```python
from build123d import *

# Parameters (mm, degrees)
CROSSRECESS_DEPTH = 0.825
DRAFT9_ANGLE      = 30
FILLET5_R         = 0.3


with BuildPart() as part:
    # Sketch1 → Base (revolve)
    with BuildSketch(Plane.XY):
        Polygon((17, 1.5), (2.65, 1.5), (1.65, 1.5), (0.55, 2.6), (0, 2.6), (0, 0), (17, 0), align=None)
    revolve(axis=Axis((4.515812911, 0, 0), (-1, 0, 0)))

    # Sketch6 → CrossRecess (cut)
    with BuildSketch(Plane(origin=(0, 0, 0), x_dir=(0, 0, -1), z_dir=(1, 0, 0))):
        Polygon((0.32, 0.32), (0.32, 1.6), (-0.32, 1.6), (-0.32, 0.32), (-1.6, 0.32), (-1.6, -0.32), (-0.32, -0.32), (-0.32, -1.6), (0.32, -1.6), (0.32, -0.32), (1.6, -0.32), (1.6, 0.32), align=None)
    extrude(amount=CROSSRECESS_DEPTH, mode=Mode.SUBTRACT)

    # Draft9
    draft9_faces = [part.faces().sort_by_distance(p)[0] for p in [
        (0.4125, 1.6, 0),
        (0.4125, 0, 1.6),
        (0.4125, -1.6, 0),
        (0.4125, 0, -1.6),
    ]]
    draft(draft9_faces, Plane(origin=(0, 2.6, 0), x_dir=(0, 0, -1), z_dir=(-1, 0, 0)), DRAFT9_ANGLE)

    # Fillet5
    fillet5_edges = [part.edges().sort_by_distance(p)[0] for p in [
        (0.4125, 0.32, 0.32),
        (0.4125, -0.32, 0.32),
        (0.4125, -0.32, -0.32),
        (0.4125, 0.32, -0.32),
    ]]
    fillet(fillet5_edges, radius=FILLET5_R)


solid = part.part
```
Could you check a few things on this model? Use its own coordinates, in mm. A direction names the side the tool comes from. Coordinates: 2 decimals unless noted, no trailing zeros. Write each loop counter-clockwise with the first axis right and the second up, starting at its lowest first coordinate (ties: lowest second). Pieces come first, ordered by that corner, then holes. Notation, with made-up numbers: (53.25, -22.5) - (91.25, -22.5) arc R16 cw to (91.25, -16.5) - close; hole circle Ø1 at (2, 67.5). An arc over 180 degrees is marked (long way). Use a Markdown table: item, result.
Q1. Please list where these lines run through material, in increasing order: L1, parallel to Y at x = 0.75, z = -0.6; L2, parallel to X at y = 1.3, z = 0.2; L3, parallel to Y at x = 12.25, z = 0.4.
Geometry check:
| item | result |
|---|---|
| L1 | y = -2.32 to -0.32, 0.32 to 2.32 |
| L2 | x = 0.52 to 17 |
| L3 | y = -1.45 to 1.45 |
Q2. Imagine slicing it at C-C (x = 2.75). List the corners of the cut face in (y, z) for me, and give its area (3 significant figures).
Geometry check:
| item | result |
|---|---|
| outline | circle Ø3 at (0, 0) |
| area | 7.07 mm2 |
Q3. Imagine slicing it at A-A (z = 0). List the corners of the cut face in (x, y) for me (3 decimals), and give its area (3 significant figures).
Geometry check:
| item | result |
|---|---|
| outline | (0, -2.6) - (0.55, -2.6) - (1.65, -1.5) - (17, -1.5) - (17, 1.5) - (1.65, 1.5) - (0.55, 2.6) - (0, 2.6) - (0, 1.6) - (0.825, 1.124) - (0.825, -1.124) - (0, -1.6) - close |
| area | 51.2 mm2 |
Q4. I'm going to push flat-ended pins straight in: pin 1 Ø3 at (x, y) = (9.5, 1.5) entering from +Z; pin 2 Ø0.9 at (x, z) = (0, 1) entering from -Y; pin 3 Ø0.9 at (x, y) = (0.5, -1) entering from -Z; pin 4 Ø1.8 at (y, z) = (-0.5, -0.5) entering from -X. Where does each tip first touch, or does it pass through?
Geometry check:
| item | result |
|---|---|
| pin 1 | stops at z = 1.5 |
| pin 2 | stops at y = -2.54 |
| pin 3 | stops at z = -2.54 |
| pin 4 | stops at x = 0 |
Q5. Thinking about a two-plate mould opening in Y: for faces 4 (the flat face through (0.4, 1, 0.32)), 5 (the cylindrical face through (0.271, -0.338, -2.578)), 6 (the flat face through (0, 1, 1)), 7 (the flat face through (0.4, -1, -0.32)), which applies, +Y half, -Y half, draft (parallel to the pull), parting line (faces both ways), or undercut?
Geometry check:
| item | result |
|---|---|
| face 4 | undercut |
| face 5 | parting line |
| face 6 | draft |
| face 7 | undercut |
Q6. Which directions (+Z, -Z, +X, -X, +Y, -Y) give clear straight access to the entire face, cutting with the end or side of a thin tool? Please do faces 1 (the flat face through (0.825, 0, 0)), 2 (the flat face through (17, 0, 0)), 3 (the cylindrical face through (9.22, -1.5, -0.07)).
Geometry check:
| item | result |
|---|---|
| face 1 | -X |
| face 2 | +Z, -Z, +X, +Y, -Y |
| face 3 | +X |
